Verification items for the finished model (mm, model axes). A direction names the side the tool comes from. Round coordinates to 2 decimals unless told otherwise and drop trailing zeros. Write each loop counter-clockwise with the first axis right and the second up, starting at its lowest first coordinate (ties: lowest second). Pieces come first, ordered by that corner, then holes. Notation, with made-up numbers: (58.5, -12) -> (90.5, -12) arc R36 cw to (90.5, 26) -> close; hole circle Ø5 at (-5, 39). An arc over 180 degrees is marked (long way). Answer as a JSON object with one key per item and string values. Group by question number.
(1) Set-up check for faces 5 (the face through (6, 6.35, -14)), 6 (the face through (6, 6.35, 41)), 7 (the face through (6, 9, -24.606)): record each of +Z, -Z, +X, -X, +Y, -Y from which the full face is reachable in a straight line by a thin tool's end or side.
(2) Sectioned sample at D-D on z = 42. Record the cut outline in (x, y).
(3) Scan lines: L1, parallel to Y at x = 5.5, z = 37; L2, parallel to Z at x = 11, y = -2. Record each from-to range of solid material in increasing order. Write a range as from..to.
(4) Sectioned sample at C-C on y = 0. Record the cut outline in (x, z).
(5) Sectioned sample at B-B on x = 1. Record the cut outline in (y, z), and give its area (3 significant figures).
(6) Draft check along Y on faces 1 (the face through (0, 0, 14)), 2 (the face through (6, 12.435, 13)), 3 (the face through (6, -6.35, 41)), 4 (the face through (6, -6.35, -14)). Enter one of: released by +Y, released by -Y, zero draft, split by the parting line, or undercut.
(7) Sectioned sample at A-A on z = 29. Record the cut outline in (x, y).
(8) Gauge pin test, flat ends, axial feed: pin 1 Ø2 at (x, y) = (4, -1.5) entering from -Z; pin 2 Ø4 at (x, y) = (5.5, 0.5) entering from +Z; pin 3 Ø3 at (x, y) = (7.5, -1.5) entering from -Z. Record the tip position at first contact, or that the pin passes through.
```python
from build123d import *

# Parameters (mm, degrees)
F1_DEPTH = 12.7


with BuildPart() as f1:
    # F0 (on Right) → F1 (new body)
    with BuildSketch(Plane.YZ):
        with BuildLine():
            Line((6.35, -24.606245), (12.435416, -24.606245))
            Line((12.435416, -24.606245), (12.435416, 51.593755))
            Line((12.435416, 51.593755), (6.35, 51.593755))
            Line((6.35, 51.593755), (6.35, 30.427093))
            ThreePointArc((6.35, 30.427093), (0, 24.077093), (-6.35, 30.427093))
            Line((-6.35, 30.427093), (-6.35, 51.593755))
            Line((-6.35, 51.593755), (-12.435416, 51.593755))
            Line((-12.435416, 51.593755), (-12.435416, -24.606245))
            Line((-12.435416, -24.606245), (-6.35, -24.606245))
            Line((-6.35, -24.606245), (-6.35, -3.439584))
            ThreePointArc((-6.35, -3.439584), (0, 2.910416), (6.35, -3.439584))
            Line((6.35, -3.439584), (6.35, -24.606245))
        make_face()
    extrude(amount=F1_DEPTH)


solid = f1.part
```
Computed values:
{
 "1": {"face 5": "-Z, +X, -X", "face 6": "+Z, +X, -X", "face 7": "-Z, +X, -X, +Y, -Y"},
 "2": {"outline": "(0, -12.44) -> (12.7, -12.44) -> (12.7, -6.35) -> (0, -6.35) -> close; (0, 6.35) -> (12.7, 6.35) -> (12.7, 12.44) -> (0, 12.44) -> close"},
 "3": {"L1": "-12.44..-6.35, 6.35..12.44", "L2": "2.59..24.4"},
 "4": {"outline": "(0, 2.91) -> (12.7, 2.91) -> (12.7, 24.08) -> (0, 24.08) -> close"},
 "5": {"outline": "(-12.44, -24.61) -> (-6.35, -24.61) -> (-6.35, -3.44) arc R6.35 cw to (6.35, -3.44) -> (6.35, -24.61) -> (12.44, -24.61) -> (12.44, 51.59) -> (6.35, 51.59) -> (6.35, 30.43) arc R6.35 cw to (-6.35, 30.43) -> (-6.35, 51.59) -> (-12.44, 51.59) -> close", "area": "1,230 mm2"},
 "6": {"face 1": "zero draft", "face 2": "released by +Y", "face 3": "undercut", "face 4": "undercut"},
 "7": {"outline": "(0, -12.44) -> (12.7, -12.44) -> (12.7, -6.19) -> (0, -6.19) -> close; (0, 6.19) -> (12.7, 6.19) -> (12.7, 12.44) -> (0, 12.44) -> close"},
 "8": {"pin 1": "z = 2.4", "pin 2": "z = 24.59", "pin 3": "z = 2.16"}
}
